Build history of the part. All positions in model axes, mm. A direction names the side the tool comes from. Coordinates: 2 decimals unless noted, no trailing zeros.
Item 1: Flat gauge pins, fed straight in: pin 1 (11 mm diameter, centred on x = 18, y = 70, fed in from +Z); pin 2 (3.5 mm diameter, centred on x = 18, y = 70, fed in from +Z); pin 3 (3.5 mm diameter, centred on x = 19, y = 69, fed in from +Z). Where does each tip first touch, or does it go through?
Item 2: Mould opens along X. For faces 4 (the face through (0, 49, 10)), 5 (the face through (16.373, 82.394, 12.852)), 6 (the face through (247, 51, 20)) say: released by +X, released by -X, zero draft, split by the parting line, or undercut.
Item 3: Drill centre lines: line 1 along Y through (x, z) = (18, 4.35); line 2 along Y through (x, z) = (18, 1.55); line 3 along X through (y, z) = (78.5, 1.25). Where is each one in solid material? Low to high.
Item 4: 3-axis set-ups, long thin cutter, end or side, ignore diameter. For faces 1 (the face through (500, 86, 10)), 2 (the face through (484, 73, 10)), 3 (the face through (21, 67, 5.5)): which of +Z, -Z, +X, -X, +Y, -Y reach the whole face in a straight line?
from build123d import *

# Parameters (mm, degrees)
SKETCH1_W           = 500
SKETCH1_H           = 100
BOSS_EXTRUDE1_DEPTH = 20
SKETCH2_R           = 3
CUT_EXTRUDE1_DEPTH  = 511.294032887
SKETCH3_R           = 12.5
CUT_EXTRUDE2_DEPTH  = 14.5
SKETCH4_R           = 3.5
CUT_EXTRUDE3_DEPTH  = 2.6
SKETCH5_R           = 1.5
CUT_EXTRUDE4_DEPTH  = 511.108076784


with BuildPart() as part:
    # Sketch1 → Boss-Extrude1 (new body)
    with BuildSketch(Plane.XY):
        with Locations((250, 50)):
            Rectangle(SKETCH1_W, SKETCH1_H)
    extrude(amount=BOSS_EXTRUDE1_DEPTH)

    # Sketch2 → Cut-Extrude1 (cut, through all)
    with BuildSketch(Plane.XY.offset(20)):
        with Locations((18, 70)):
            Circle(SKETCH2_R)
        with BuildLine():
            Line((468, 73), (520, 73))
            ThreePointArc((520, 73), (523, 70), (520, 67))
            Line((520, 67), (468, 67))
            ThreePointArc((468, 67), (465, 70), (468, 73))
        make_face()
    extrude(amount=-CUT_EXTRUDE1_DEPTH, mode=Mode.SUBTRACT)

    # Sketch3 → Cut-Extrude2 (cut)
    with BuildSketch(Plane.XY.offset(20)):
        with Locations((18, 70)):
            Circle(SKETCH3_R)
    extrude(amount=-CUT_EXTRUDE2_DEPTH, mode=Mode.SUBTRACT)

    # Sketch4 → Cut-Extrude3 (cut)
    with BuildSketch(Plane.XY.offset(5.5)):
        with Locations((18, 70)):
            Circle(SKETCH4_R)
    extrude(amount=-CUT_EXTRUDE3_DEPTH, mode=Mode.SUBTRACT)

    # Sketch5 → Cut-Extrude4 (cut, through all)
    with BuildSketch(Plane.XY.offset(5.5)):
        with Locations((18, 61.5)):
            Circle(SKETCH5_R)
        with Locations((18, 78.5)):
            Circle(SKETCH5_R)
    extrude(amount=-CUT_EXTRUDE4_DEPTH, mode=Mode.SUBTRACT)


solid = part.part
Filled sheet:
1. pin 1: stops at z = 5.5
1. pin 2: passes through
1. pin 3: stops at z = 2.9
2. face 4: released by -X
2. face 5: undercut
2. face 6: zero draft
3. line 1: y = 0 to 60, 63 to 66.5, 73.5 to 77, 80 to 100
3. line 2: y = 0 to 60, 63 to 67, 73 to 77, 80 to 100
3. line 3: x = 0 to 16.5, 19.5 to 500
4. face 1: +Z, -Z, +X, +Y, -Y
4. face 2: +Z, -Z, +X
4. face 3: +Z
